Geometry: final body of the model. Coordinates: model frame, mm. A direction names the side the tool comes from. Round coordinates to 2 decimals unless told otherwise and drop trailing zeros. Write each loop counter-clockwise with the first axis right and the second up, starting at its lowest first coordinate (ties: lowest second). Pieces come first, ordered by that corner, then holes. Notation, with made-up numbers: (49.5, -16.75) - (77.5, -16.75) arc R16 ccw to (77.5, 1.25) - close; hole circle Ø10 at (13, 28). An arc over 180 degrees is marked (long way). Write each question's results on one line, items separated by ' | '.
from build123d import *

# Parameters (mm, degrees)
SKETCH1_W           = 55
SKETCH1_H           = 20
BOSS_EXTRUDE1_DEPTH = 2
SKETCH2_W           = 2
SKETCH2_H           = 20
BOSS_EXTRUDE2_DEPTH = 37
SKETCH3_R           = 5
CUT_EXTRUDE1_DEPTH  = 56
CUT_EXTRUDE2_DEPTH  = 56
SKETCH5_R           = 1.5
CUT_EXTRUDE3_DEPTH  = 40


with BuildPart() as part:
    # Sketch1 → Boss-Extrude1 (new body)
    with BuildSketch(Plane(origin=(0, 0, 0), x_dir=(1, 0, 0), z_dir=(0, 1, 0))):
        Rectangle(SKETCH1_W, SKETCH1_H)
    extrude(amount=-BOSS_EXTRUDE1_DEPTH)

    # Sketch2 → Boss-Extrude2 (add)
    with BuildSketch(Plane.XZ.offset(2)):
        with Locations((-26.5, 0)):
            Rectangle(SKETCH2_W, SKETCH2_H)
        with Locations((26.5, 0)):
            Rectangle(SKETCH2_W, SKETCH2_H)
    extrude(amount=BOSS_EXTRUDE2_DEPTH)

    # Sketch3 → Cut-Extrude1 (cut, through all)
    with BuildSketch(Plane(origin=(27.5, 0, 0), x_dir=(0, 0, -1), z_dir=(1, 0, 0))):
        with Locations((0, -30)):
            Circle(SKETCH3_R)
    extrude(amount=-CUT_EXTRUDE1_DEPTH, mode=Mode.SUBTRACT)

    # Sketch4 → Cut-Extrude2 (cut, through all)
    with BuildSketch(Plane.ZY.offset(27.5)):
        with BuildLine():
            ThreePointArc((0, -39), (-7.071067812, -36.071067812), (-10, -29))
            Line((-10, -29), (-10, -39))
            Line((-10, -39), (0, -39))
        make_face()
        with BuildLine():
            Line((10, -39), (10, -29))
            ThreePointArc((10, -29), (7.071067812, -36.071067812), (0, -39))
            Line((0, -39), (10, -39))
        make_face()
    extrude(amount=-CUT_EXTRUDE2_DEPTH, mode=Mode.SUBTRACT)

    # Sketch5 → Cut-Extrude3 (cut, through all)
    with BuildSketch(Plane(origin=(0, 0, 0), x_dir=(1, 0, 0), z_dir=(0, 1, 0))):
        with Locations((5, 5)):
            Circle(SKETCH5_R)
        with Locations((15, 5)):
            Circle(SKETCH5_R)
        with Locations((-15, 5)):
            Circle(SKETCH5_R)
        with Locations((-5, 5)):
            Circle(SKETCH5_R)
    extrude(amount=-CUT_EXTRUDE3_DEPTH, mode=Mode.SUBTRACT)


solid = part.part
Q1. Section query B-B, the plane y = -26. Return loops of the section in (x, z).
Answer block:
outline: (-27.5, -10) - (-25.5, -10) - (-25.5, -3) - (-27.5, -3) - close; (-27.5, 3) - (-25.5, 3) - (-25.5, 10) - (-27.5, 10) - close; (25.5, -10) - (27.5, -10) - (27.5, -3) - (25.5, -3) - close; (25.5, 3) - (27.5, 3) - (27.5, 10) - (25.5, 10) - close
Q2. Ray query, line 1 along X through (y, z) = (-0.95, -5); line 2 along X through (y, z) = (-16, 0.5); line 3 along Y through (x, z) = (26.9, 0). Return the intervals inside material, ascending.
Answer block:
line 1: -27.5 to -16.5, -13.5 to -6.5, -3.5 to 3.5, 6.5 to 13.5, 16.5 to 27.5 | line 2: -27.5 to -25.5, 25.5 to 27.5 | line 3: -39 to -35, -25 to 0
Q3. Section query C-C, the plane y = -20. Return loops of the section in (x, z).
Answer block:
outline: (-27.5, -10) - (-25.5, -10) - (-25.5, 10) - (-27.5, 10) - close; (25.5, -10) - (27.5, -10) - (27.5, 10) - (25.5, 10) - close
Q4. Mould query, pull axis X, two halves, no side actions, for faces 1 (the cylindrical face through (-26.49, -34.88, 1.08)), 2 (the flat face through (27.5, -19, 0)), 3 (the flat face through (-25.5, -16, 0)). Classes: pulls with the +X half, pulls with the -X half, needs draft (parallel to the pull), parting line crosses it, or undercut.
Answer block:
face 1: needs draft | face 2: pulls with the +X half | face 3: undercut
Q5. Pin query (flat end, axial travel): pin 1 (2.5 mm diameter, centred on x = -5, z = -5, fed in from +Y); pin 2 (6 mm diameter, centred on x = -9, z = -4.5, fed in from -Y). Return the tip coordinate at first contact, or that it passes through.
Answer block:
pin 1: through | pin 2: y = -2
Q6. Access query for faces 4 (the cylindrical face through (13.5, -0.99, -5.07)), 5 (the flat face through (25.5, -16, 0)). Directions: +Z, -Z, +X, -X, +Y, -Y. A direction counts if a zero-diameter tool reaches every point of the face in a straight line with its end or side. Return the directions, or none.
Answer block:
face 4: +Y, -Y | face 5: +Z, -Z, -Y
Q7. Section query D-D, the plane z = 2.25. Return loops of the section in (x, y), plus the area to 3 significant figures.
Answer block:
outline: (-27.5, -38.74) - (-25.5, -38.74) - (-25.5, -34.47) - (-27.5, -34.47) - close; (-27.5, -25.53) - (-25.5, -25.53) - (-25.5, -2) - (25.5, -2) - (25.5, -25.53) - (27.5, -25.53) - (27.5, 0) - (-27.5, 0) - close; (25.5, -38.74) - (27.5, -38.74) - (27.5, -34.47) - (25.5, -34.47) - close | area: 221 mm2
Q8. Section query A-A, the plane x = -5. Return loops of the section in (y, z).
Answer block:
outline: (-2, -10) - (0, -10) - (0, -6.5) - (-2, -6.5) - close; (-2, -3.5) - (0, -3.5) - (0, 10) - (-2, 10) - close
